```python
from build123d import *

# Parameters (mm, degrees)
SALIENTE_EXTRUIR1_DEPTH = 10
CROQUIS7_W              = 86.1
CROQUIS7_H              = 2
CORTAR_EXTRUIR4_DEPTH   = 3
CROQUIS15_R             = 1.435
CORTAR_EXTRUIR10_DEPTH  = 10
CROQUIS16_W             = 10
CROQUIS16_H             = 10
SALIENTE_EXTRUIR7_DEPTH = 10
CROQUIS17_W             = 3
CROQUIS17_H             = 2
CORTAR_EXTRUIR11_DEPTH  = 3
CROQUIS18_R             = 1.435
CORTAR_EXTRUIR12_DEPTH  = 10
CROQUIS19_R             = 1.435
CORTAR_EXTRUIR13_DEPTH  = 10
CROQUIS20_R             = 1.435
CORTAR_EXTRUIR14_DEPTH  = 10
CROQUIS21_R             = 2.435
CORTAR_EXTRUIR15_DEPTH  = 10
CROQUIS2_W              = 16
CROQUIS2_H              = 16
CORTAR_EXTRUIR16_DEPTH  = 3
CROQUIS22_R             = 1.435
CORTAR_EXTRUIR17_DEPTH  = 10


with BuildPart() as part:
    # Croquis1 → Saliente-Extruir1 (new body)
    with BuildSketch(Plane(origin=(0, 0, 0), x_dir=(1, 0, 0), z_dir=(0, 1, 0))):
        Polygon((22.5, -35), (51.5, -35), (51.5, 35), (22.5, 35), (-22.5, 35), (-34.6, 35), (-34.6, -35), (-22.5, -35), align=None)
    extrude(amount=SALIENTE_EXTRUIR1_DEPTH)

    # Croquis7 → Cortar-Extruir4 (cut)
    with BuildSketch(Plane(origin=(0, 10, 0), x_dir=(1, 0, 0), z_dir=(0, 1, 0))):
        with Locations((8.45, 31)):
            Rectangle(CROQUIS7_W, CROQUIS7_H)
    cortar_extruir4 = extrude(amount=-CORTAR_EXTRUIR4_DEPTH, mode=Mode.SUBTRACT)

    # Simetría2: Cortar-Extruir4 across plane
    add(cortar_extruir4.mirror(Plane.XY), mode=Mode.SUBTRACT)

    # Croquis15 → Cortar-Extruir10 (cut)
    with BuildSketch(Plane(origin=(0, 10, 0), x_dir=(1, 0, 0), z_dir=(0, 1, 0))):
        with Locations((-31.1, -15)):
            Circle(CROQUIS15_R)
    cortar_extruir10 = extrude(amount=-CORTAR_EXTRUIR10_DEPTH, mode=Mode.SUBTRACT)

    # Simetría4: Cortar-Extruir10 across plane
    add(cortar_extruir10.mirror(Plane.XY), mode=Mode.SUBTRACT)

    # Croquis16 → Saliente-Extruir7 (add)
    with BuildSketch(Plane(origin=(51.5, 0, 0), x_dir=(0, 0, -1), z_dir=(1, 0, 0))):
        with Locations((-30, 5)):
            Rectangle(CROQUIS16_W, CROQUIS16_H)
    saliente_extruir7 = extrude(amount=SALIENTE_EXTRUIR7_DEPTH)

    # Croquis17 → Cortar-Extruir11 (cut)
    with BuildSketch(Plane(origin=(0, 10, 0), x_dir=(1, 0, 0), z_dir=(0, 1, 0))):
        with Locations((53, -31)):
            Rectangle(CROQUIS17_W, CROQUIS17_H)
    cortar_extruir11 = extrude(amount=-CORTAR_EXTRUIR11_DEPTH, mode=Mode.SUBTRACT)

    # Simetría5: Saliente-Extruir7, Cortar-Extruir11 across plane
    add(saliente_extruir7.mirror(Plane.XY))
    add(cortar_extruir11.mirror(Plane.XY), mode=Mode.SUBTRACT)

    # Croquis18 → Cortar-Extruir12 (cut)
    with BuildSketch(Plane(origin=(0, 10, 0), x_dir=(1, 0, 0), z_dir=(0, 1, 0))):
        with Locations((48, 15)):
            Circle(CROQUIS18_R)
    cortar_extruir12 = extrude(amount=-CORTAR_EXTRUIR12_DEPTH, mode=Mode.SUBTRACT)

    # Simetría6: Cortar-Extruir12 across plane
    add(cortar_extruir12.mirror(Plane.XY), mode=Mode.SUBTRACT)

    # Croquis19 → Cortar-Extruir13 (cut)
    with BuildSketch(Plane.ZY.offset(34.6)):
        with Locations((26.5, 5)):
            Circle(CROQUIS19_R)
    cortar_extruir13 = extrude(amount=-CORTAR_EXTRUIR13_DEPTH, mode=Mode.SUBTRACT)

    # Simetría7: Cortar-Extruir13 across plane
    add(cortar_extruir13.mirror(Plane.XY), mode=Mode.SUBTRACT)

    # Croquis20 → Cortar-Extruir14 (cut)
    with BuildSketch(Plane.XY.offset(35)):
        with Locations((56.5, 5)):
            Circle(CROQUIS20_R)
    cortar_extruir14 = extrude(amount=-CORTAR_EXTRUIR14_DEPTH, mode=Mode.SUBTRACT)

    # Simetría8: Cortar-Extruir14 across plane
    add(cortar_extruir14.mirror(Plane.XY), mode=Mode.SUBTRACT)

    # Croquis21 → Cortar-Extruir15 (cut)
    with BuildSketch(Plane.XZ):
        with Locations((13.45, 0)):
            Circle(CROQUIS21_R)
        with Locations((43.45, 0)):
            Circle(CROQUIS21_R)
        with Locations((-29.05, 0)):
            Circle(CROQUIS21_R)
    extrude(amount=-CORTAR_EXTRUIR15_DEPTH, mode=Mode.SUBTRACT)

    # Croquis2 → Cortar-Extruir16 (cut)
    with BuildSketch(Plane(origin=(0, 10, 0), x_dir=(1, 0, 0), z_dir=(0, 1, 0))):
        with Locations((9.5, 0)):
            Rectangle(CROQUIS2_W, CROQUIS2_H)
    cortar_extruir16 = extrude(amount=-CORTAR_EXTRUIR16_DEPTH, mode=Mode.SUBTRACT)

    # Simetría9: Cortar-Extruir16 across plane
    add(cortar_extruir16.mirror(Plane(origin=(0, 0, 0), x_dir=(0, 0, 1), z_dir=(1, 0, 0))), mode=Mode.SUBTRACT)

    # Croquis22 → Cortar-Extruir17 (cut)
    with BuildSketch(Plane(origin=(0, 10, 0), x_dir=(1, 0, 0), z_dir=(0, 1, 0))):
        with Locations((-9.5, 11.5)):
            Circle(CROQUIS22_R)
        with Locations((-21, 0)):
            Circle(CROQUIS22_R)
        with Locations((-9.5, -11.5)):
            Circle(CROQUIS22_R)
    cortar_extruir17 = extrude(amount=-CORTAR_EXTRUIR17_DEPTH, mode=Mode.SUBTRACT)

    # Simetría10: Cortar-Extruir17 across plane
    add(cortar_extruir17.mirror(Plane(origin=(0, 0, 0), x_dir=(0, 0, 1), z_dir=(1, 0, 0))), mode=Mode.SUBTRACT)


solid = part.part
```
Work out the finished part from the listing and answer in its coordinate system (mm). A direction names the side the tool comes from. Round coordinates to 2 decimals unless told otherwise and drop trailing zeros. Loops run counter-clockwise (first coordinate to the right, second up) from the corner with the lowest first, then second, coordinate; pieces in that order, holes last. Notation, with made-up numbers: M 4.5,-15.5 L 30.5,-15.5 A16 cw 30.5,-1.5 Z; hole C 6,3 d6. An arc over 180 degrees is marked long. Use CSV: the item, a comma, the result in double quotes.
Q1. Each of these flat-tipped pins is pushed along its axis until it touches: pin 1 (1.6 mm diameter, centred on x = 27.5, z = -31, fed in from +Y); pin 2 (3.5 mm diameter, centred on x = -31.1, z = 15, fed in from -Y); pin 3 (1.5 mm diameter, centred on y = 2.5, z = 8, fed in from +X). Where does it stop, or does it pass through?
Determined:
pin 1,"y = 7"
pin 2,"y = 0"
pin 3,"x = 51.5"
Q2. Section B-B, the plane z = 11.5 is taken. Determine the outline of the cut face in (x, y) (3 decimals), then the cut area to 3 significant figures.
Determined:
outline,"M -34.6,0 L -10.935,0 L -10.935,10 L -34.6,10 Z; M -8.065,0 L 8.065,0 L 8.065,10 L -8.065,10 Z; M 10.935,0 L 51.5,0 L 51.5,10 L 10.935,10 Z"
area,"804 mm2"
Q3. Section A-A, the plane x = 43.45 is taken. Determine the outline of the cut face in (y, z) (3 decimals).
Determined:
outline,"M 0,-35 L 10,-35 L 10,-32 L 7,-32 L 7,-30 L 10,-30 L 10,-2.435 L 0,-2.435 Z; M 0,2.435 L 10,2.435 L 10,30 L 7,30 L 7,32 L 10,32 L 10,35 L 0,35 Z"
Q4. The mould has two halves that part along Z. Classify faces 5 (the cylindrical face through (-19.674, 5.07, 0.55)), 6 (the flat face through (13, 5, 35)), 7 (the flat face through (9, 7, -31)), 8 (the cylindrical face through (57.826, 4.45, -30.07)): pulls with the +Z half, pulls with the -Z half, needs draft (parallel to the pull), parting line crosses it, or undercut.
Determined:
face 5,"undercut"
face 6,"pulls with the +Z half"
face 7,"undercut"
face 8,"needs draft"
Q5. Section C-C, the plane x = -3.5 is taken. Determine the outline of the cut face in (y, z), then the cut area to 3 significant figures.
Determined:
outline,"M 0,-35 L 10,-35 L 10,-32 L 7,-32 L 7,-30 L 10,-30 L 10,-8 L 7,-8 L 7,8 L 10,8 L 10,30 L 7,30 L 7,32 L 10,32 L 10,35 L 0,35 Z"
area,"640 mm2"
Q6. Section D-D, the plane z = -26.5 is taken. Determine the outline of the cut face in (x, y) (3 decimals), then the cut area to 3 significant figures.
Determined:
outline,"M -34.6,0 L 61.5,0 L 61.5,10 L -34.6,10 L -34.6,6.435 L -24.6,6.435 L -24.6,3.565 L -34.6,3.565 Z; hole C 56.5,5 d2.87"
area,"926 mm2"
Q7. Consider L1, parallel to X at y = 7.25, z = -6; L2, parallel to X at y = 5.5, z = -11.5 (3 decimals); L3, parallel to Z at x = 9.5, y = 3.5 (3 decimals). Determine where each line is inside the solid, lowest interval first.
Determined:
L1,"-34.6 to -17.5, -1.5 to 1.5, 17.5 to 51.5"
L2,"-34.6 to -10.935, -8.065 to 8.065, 10.935 to 51.5"
L3,"-35 to -12.935, -10.065 to 10.065, 12.935 to 35"
Q8. A tool of negligible diameter and unlimited length cuts with its end or side. For faces 1 (the flat face through (51.5, 5, 0)), 2 (the flat face through (54.5, 9, -31)), 3 (the flat face through (-24.6, 5, 26)), 4 (the flat face through (9, 9, -8)), from which of +Z, -Z, +X, -X, +Y, -Y can it reach the whole face along a straight path? Write none if from no direction.
Determined:
face 1,"+X, +Y, -Y"
face 2,"-X, +Y"
face 3,"-X"
face 4,"+Y"
